from build123d import *

# Parameters (mm, degrees)
F0_R     = 158.75
F0_R_2   = 11.1125
F1_DEPTH = 36.4236
F2_R     = 114.99977
F2_R_2   = 101.6
F3_DEPTH = 6.35
F2_R_3   = 51.59375
F4_DEPTH = 8.255
F5_DEPTH = 36.4236


with BuildPart() as f1:
    # F0 (on Front) → F1 (new body)
    with BuildSketch(Plane.XZ):
        Circle(F0_R)
        with Locations((-67.46875, -116.859303)):
            Circle(F0_R_2, mode=Mode.SUBTRACT)
        with Locations((-116.859303, -67.46875)):
            Circle(F0_R_2, mode=Mode.SUBTRACT)
        with Locations((0, -134.9375)):
            Circle(F0_R_2, mode=Mode.SUBTRACT)
        with Locations((67.46875, -116.859303)):
            Circle(F0_R_2, mode=Mode.SUBTRACT)
        with Locations((116.859303, -67.46875)):
            Circle(F0_R_2, mode=Mode.SUBTRACT)
        with Locations((-134.9375, 0)):
            Circle(F0_R_2, mode=Mode.SUBTRACT)
        with Locations((-116.859303, 67.46875)):
            Circle(F0_R_2, mode=Mode.SUBTRACT)
        with Locations((-67.46875, 116.859303)):
            Circle(F0_R_2, mode=Mode.SUBTRACT)
        with Locations((134.9375, 0)):
            Circle(F0_R_2, mode=Mode.SUBTRACT)
        with Locations((116.859303, 67.46875)):
            Circle(F0_R_2, mode=Mode.SUBTRACT)
        with Locations((67.46875, 116.859303)):
            Circle(F0_R_2, mode=Mode.SUBTRACT)
        with Locations((0, 134.9375)):
            Circle(F0_R_2, mode=Mode.SUBTRACT)
    extrude(amount=F1_DEPTH)

    # F2 (on face) → F3 (cut)
    with BuildSketch(Plane.XZ):
        Circle(F2_R)
        Circle(F2_R_2, mode=Mode.SUBTRACT)
    extrude(amount=F3_DEPTH, mode=Mode.SUBTRACT)

    # F2 (on face) → F4 (cut)
    with BuildSketch(Plane.XZ):
        Circle(F2_R_2)
        Circle(F2_R_3, mode=Mode.SUBTRACT)
    extrude(amount=F4_DEPTH, mode=Mode.SUBTRACT)

    # F2 (on face) → F5 (cut)
    with BuildSketch(Plane.XZ):
        Circle(F2_R_3)
    extrude(amount=F5_DEPTH, mode=Mode.SUBTRACT)


solid = f1.part
Could you check a few things on this model? Use its own coordinates, in mm. A direction names the side the tool comes from. Coordinates: 2 decimals unless noted, no trailing zeros. Write each loop counter-clockwise with the first axis right and the second up, starting at its lowest first coordinate (ties: lowest second). Pieces come first, ordered by that corner, then holes. Notation, with made-up numbers: M 3.25,65.5 L 20.25,65.5 A16 ccw 20.25,93.5 Z; hole C 81,5 d7. An arc over 180 degrees is marked long. One line per question, with ' | ' between items.
1) Imagine slicing it at B-B, the plane z = 0. Write out the boundary of the cut face in (x, y) (3 decimals), and give its area (3 significant figures).
Checks:
outline: M -158.75,-36.424 L -146.05,-36.424 L -146.05,0 L -158.75,0 Z; M -123.825,-36.424 L -51.594,-36.424 L -51.594,-8.255 L -101.6,-8.255 L -101.6,-6.35 L -115,-6.35 L -115,0 L -123.825,0 Z; M 51.594,-36.424 L 123.825,-36.424 L 123.825,0 L 115,0 L 115,-6.35 L 101.6,-6.35 L 101.6,-8.255 L 51.594,-8.255 Z; M 146.05,-36.424 L 158.75,-36.424 L 158.75,0 L 146.05,0 Z | area: 5,190 mm²
2) Imagine slicing it at A-A, the plane x = 0. Write out the boundary of the cut face in (y, z) (3 decimals), and give its area (3 significant figures).
Checks:
outline: M -36.424,-158.75 L 0,-158.75 L 0,-146.05 L -36.424,-146.05 Z; M -36.424,-123.825 L 0,-123.825 L 0,-115 L -6.35,-115 L -6.35,-101.6 L -8.255,-101.6 L -8.255,-51.594 L -36.424,-51.594 Z; M -36.424,51.594 L -8.255,51.594 L -8.255,101.6 L -6.35,101.6 L -6.35,115 L 0,115 L 0,123.825 L -36.424,123.825 Z; M -36.424,146.05 L 0,146.05 L 0,158.75 L -36.424,158.75 Z | area: 5,190 mm²
3) If we mould it in two halves opening along Z, with no side actions, what happens to faces 1 (the face through (151.42, -17.96, 47.68)), 2 (the face through (-2.41, -17.96, 124.09)), 3 (the face through (68, -36.424, 2))? For each: released by +Z, released by -Z, zero draft, split by the parting line, or undercut.
Checks:
face 1: split by the parting line | face 2: undercut | face 3: zero draft
4) I need wall thicknesses on probe 1 along Z at (x, y) = (-115.5, -22); probe 2 along Z at (x, y) = (74, -6.5); probe 3 along Z at (x, y) = (67, -32). Which ranges of each line are inside material? Lowest first, please. Write a range as [from, to].
Checks:
probe 1: [-108.91, -78.5], [-56.44, 56.44], [78.5, 108.91] | probe 2: [-140.45, -125.85], [-107.87, -69.62], [69.62, 107.87], [125.85, 140.45] | probe 3: [-143.92, -127.96], [-105.76, 105.76], [127.96, 143.92]
5) Imagine slicing it at D-D, the plane z = 47.5. Write out the boundary of the cut face in (x, y) (3 decimals).
Checks:
outline: M -151.477,-36.424 L -20.141,-36.424 L -20.141,-8.255 L -89.813,-8.255 L -89.813,-6.35 L -104.732,-6.35 L -104.732,0 L -151.477,0 Z; M 20.141,-36.424 L 151.477,-36.424 L 151.477,0 L 104.732,0 L 104.732,-6.35 L 89.813,-6.35 L 89.813,-8.255 L 20.141,-8.255 Z
6) For faces 4 (the face through (-106.6, -18, 63.2)), 5 (the face through (-47, -8.255, 24)), which set-ups out of +Z, -Z, +X, -X, +Y, -Y let a thin tool reach every point of the face, with its end or its side?
Checks:
face 4: +Y, -Y | face 5: +Y
7) Imagine slicing it at C-C, the plane x = 133.5. Write out the boundary of the cut face in (y, z).
Checks:
outline: M -36.42,-85.9 L 0,-85.9 L 0,-11.02 L -36.42,-11.02 Z; M -36.42,11.02 L 0,11.02 L 0,85.9 L -36.42,85.9 Z
8) For pin 1 Ø4 at (y, z) = (-23.5, 12.5) entering from -X; pin 2 Ø1 at (x, y) = (-126.5, -22) entering from -Z; pin 3 Ø10 at (x, y) = (48, -21) entering from +Z, each with a flat end and sliding along its axis, tell me the tip position at first contact or that it passes through.
Checks:
pin 1: x = -158.4 | pin 2: z = -96.57 | pin 3: z = 152.82
